from build123d import *

# Parameters (mm, degrees)
BOSS_EXTRU_1_DEPTH = 15
ESQUISSE2_R        = 6
BOSS_EXTRU_2_DEPTH = 5
CONG_1_R           = 5
CONG_2_R           = 2


with BuildPart() as part:
    # Esquisse1 → Boss.-Extru.1 (new body)
    with BuildSketch(Plane(origin=(0, 0, 0), x_dir=(1, 0, 0), z_dir=(0, 1, 0))):
        with BuildLine():
            ThreePointArc((28.831406487, 15), (27.338937497, 17.573630715), (25.617376915, 20))
            ThreePointArc((25.617376915, 20), (-32.5, 0), (25.617376915, -20))
            ThreePointArc((25.617376915, -20), (27.338937497, -17.573630715), (28.831406487, -15))
            Line((28.831406487, -15), (23.048861143, -15))
            ThreePointArc((23.048861143, -15), (-27.5, 0), (23.048861143, 15))
            Line((23.048861143, 15), (28.831406487, 15))
        make_face()
        with BuildLine():
            Line((42.5, 20), (25.617376915, 20))
            ThreePointArc((25.617376915, 20), (27.338937497, 17.573630715), (28.831406487, 15))
            Line((28.831406487, 15), (37.5, 15))
            Line((37.5, 15), (37.5, -15))
            Line((37.5, -15), (28.831406487, -15))
            ThreePointArc((28.831406487, -15), (27.338937497, -17.573630715), (25.617376915, -20))
            Line((25.617376915, -20), (42.5, -20))
            Line((42.5, -20), (42.5, 20))
        make_face()
    extrude(amount=BOSS_EXTRU_1_DEPTH)

    # Esquisse2 → Boss.-Extru.2 (add)
    with BuildSketch(Plane(origin=(0, 15, 0), x_dir=(1, 0, 0), z_dir=(0, 1, 0))):
        with BuildLine():
            Line((42.5, 20), (25.617376915, 20))
            ThreePointArc((25.617376915, 20), (-32.5, 0), (25.617376915, -20))
            Line((25.617376915, -20), (42.5, -20))
            Line((42.5, -20), (42.5, 20))
        make_face()
        with Locations((30, 0)):
            Circle(ESQUISSE2_R, mode=Mode.SUBTRACT)
    extrude(amount=BOSS_EXTRU_2_DEPTH)

    # Congé1
    cong_1_edges = [part.edges().sort_by_distance(p)[0] for p in [
        (42.5, 20, 0),
        (34.058688457, 20, -20),
        (-32.5, 20, 0),
        (34.058688457, 20, 20),
    ]]
    fillet(cong_1_edges, radius=CONG_1_R)

    # Congé2
    cong_2_edges = [part.edges().sort_by_distance(p)[0] for p in [
        (-27.5, 0, 0),
        (30.274430572, 0, 15),
        (37.5, 0, 0),
        (30.274430572, 0, -15),
        (42.5, 0, 0),
        (34.058688457, 0, 20),
        (-32.5, 0, 0),
        (34.058688457, 0, -20),
    ]]
    fillet(cong_2_edges, radius=CONG_2_R)


solid = part.part
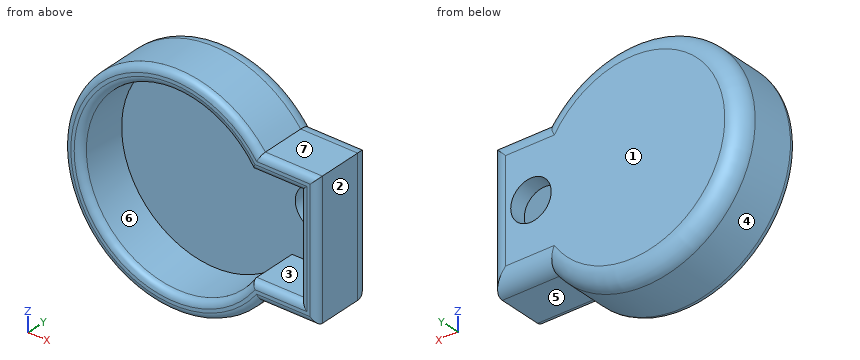
Geometry check sheet. Reference: the model listing, model coordinates, mm. Face numbers are marked on the shaded views. A direction names the side the tool comes from. Round coordinates to 2 decimals unless told otherwise and drop trailing zeros. Order: outer loops, then holes, each group sorted by start corner. A loop starts at its lowest first (then second) coordinate and runs counter-clockwise, first axis right, second up. Notation, with made-up numbers: M -9,43 L 33,43 A24 cw 33,53 Z; hole C 27.25,15.5 d2. An arc over 180 degrees is marked long. Answer in a Markdown table with one row per item. Add a question column.
Item 1: Sectioned sample at B-B, the plane z = 0. Enter the section's corners in (x, y), plus the area to 3 significant figures.
Item 2: Depth check by flat-ended pin: pin 1 Ø10.5 at (x, y) = (30, 7) entering from +Z; pin 2 Ø12 at (y, z) = (15, -14.5) entering from -X; pin 3 Ø2 at (x, y) = (12, 6) entering from +Z. Enter the tip coordinate at first touch or a pass-through.
Item 3: Sectioned sample at A-A, the plane x = 30. Enter the section's corners in (y, z).
Item 4: Draft check along X on the marked faces 1, 2, 3 and 4. Enter one of: released by +X, released by -X, zero draft, split by the parting line, or undercut.
Item 5: Sectioned sample at C-C, the plane y = 8. Enter the section's corners in (x, z).
Item 6: Set-up check for the marked faces 5, 6 and 7: record each of +Z, -Z, +X, -X, +Y, -Y from which the full face is reachable in a straight line by a thin tool's end or side.
Item 7: Sectioned sample at D-D, the plane y = 18.75. Enter the section's corners in (x, z), plus the area to 3 significant figures.
Item 8: Material ranges on L1, parallel to X at y = 6, z = 0; L2, parallel to Z at x = 0, y = 10; L3, parallel to Y at x = 5, z = 16.5, recorded low to high. Write a range as [from, to].
Filled in:
| question | item | result |
|---|---|---|
| 1 | outline | M -32.5,2 A2 ccw -30.5,0 L -29.5,0 A2 ccw -27.5,2 L -27.5,15 L 24,15 L 24,20 L -27.5,20 A5 ccw -32.5,15 Z; M 36,15 L 37.5,15 L 37.5,2 A2 ccw 39.5,0 L 40.5,0 A2 ccw 42.5,2 L 42.5,15 A5 ccw 37.5,20 L 36,20 Z |
| 1 | area | 451 mm² |
| 2 | pin 1 | stops at z = 21.06 |
| 2 | pin 2 | stops at x = -31.37 |
| 2 | pin 3 | stops at z = 30.58 |
| 3 | outline | M 0,-18 A2 ccw 2,-20 L 15,-20 A5 ccw 20,-15 L 20,-6 L 15,-6 L 15,-15 L 2,-15 A2 ccw 0,-17 Z; M 0,17 A2 ccw 2,15 L 15,15 L 15,6 L 20,6 L 20,15 A5 ccw 15,20 L 2,20 A2 ccw 0,18 Z |
| 4 | face 1 | zero draft |
| 4 | face 2 | released by +X |
| 4 | face 3 | undercut |
| 4 | face 4 | split by the parting line |
| 5 | outline | M 25.62,-20 L 42.5,-20 L 42.5,20 L 25.62,20 A32.5 ccw long Z; hole M 23.05,-15 L 37.5,-15 L 37.5,15 L 23.05,15 A27.5 ccw long Z |
| 6 | face 5 | -Z, +X, +Y, -Y |
| 6 | face 6 | -Y |
| 6 | face 7 | +Z, +X, +Y, -Y |
| 7 | outline | M 24.78,-18.31 L 40.81,-18.31 L 40.81,18.31 L 24.78,18.31 A30.81 ccw long Z; hole C 30,0 d12 |
| 7 | area | 3,310 mm² |
| 8 | L1 | x = [-32.5, -27.5], [37.5, 42.5] |
| 8 | L2 | z = [-32.5, -27.5], [27.5, 32.5] |
| 8 | L3 | y = [15, 20] |
